Check sheet for the drawn part. Datum: minimum x, y, z corner. Units: mm. Give positions to 0.01 mm unless a question says otherwise; leave off trailing zeros. Write each loop counter-clockwise with the first axis right and the second up, starting at its lowest first coordinate (ties: lowest second). Pieces come first, ordered by that corner, then holes. Notation, with made-up numbers: (65.5, -22) - (115.5, -22) arc R15 cw to (115.5, -6) - close; hole circle Ø6 at (-31.5, -17). An arc over 180 degrees is marked (long way). Use a Markdown table: item, result.
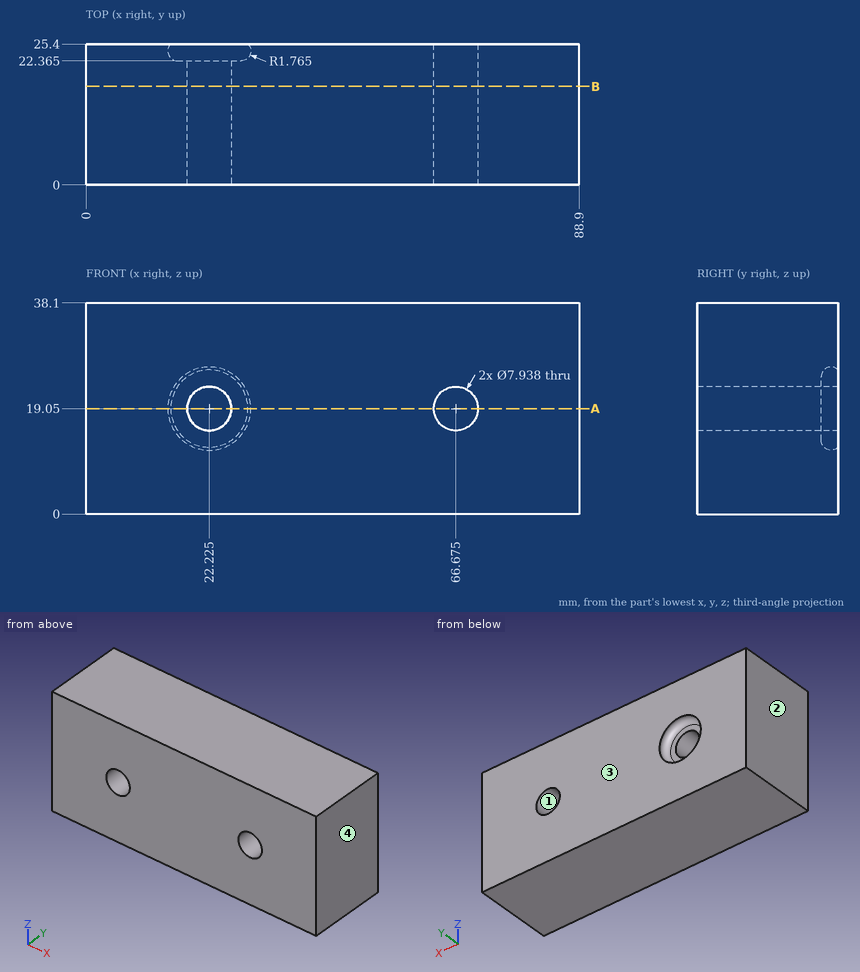
1) Section check B-B on y = 17.75. Count the separate pieces of the cut face and the enclosed holes in it, then the cut area to 3 significant figures.
Working result:
| item | result |
|---|---|
| separate pieces | 1 |
| enclosed holes | 2 |
| area | 3,290 mm² |
2) Material ranges on L1, parallel to X at y = 10.5, z = 15.5; L2, parallel to X at y = 8, z = 17 (1 decimal); L3, parallel to Z at x = 68.5, y = 15.75 (1 decimal), recorded low to high. Write a range as from..to.
Working result:
| item | result |
|---|---|
| L1 | x = 0..20.45, 24..64.9, 68.45..88.9 |
| L2 | x = 0..18.8, 25.6..63.3, 70.1..88.9 |
| L3 | z = 0..15.5, 22.6..38.1 |
3) Section check A-A on z = 19.05. Record the boundary of the cut face in (x, y) (1 decimal), then the cut area to 4 significant figures.
Working result:
| item | result |
|---|---|
| outline | (0, 0) - (18.3, 0) - (18.3, 22.4) - (16.5, 22.4) arc R1.8 cw to (15.3, 25.4) - (0, 25.4) - close; (26.2, 0) - (62.7, 0) - (62.7, 25.4) - (29.2, 25.4) arc R1.8 cw to (28, 22.4) - (26.2, 22.4) - close; (70.6, 0) - (88.9, 0) - (88.9, 25.4) - (70.6, 25.4) - close |
| area | 1,835 mm² |
4) Depth check by flat-ended pin: P1, Ø7, axis at x = 22.225, z = 19.05, coming from the +Y side. Enter the tip coordinate at first touch or a pass-through.
Working result:
| item | result |
|---|---|
| P1 | passes through |
5) Mould release check, pull along X, two halves, no side actions. Record for the marked faces 1, 2, 3 and 4: pulls with the +X half, pulls with the -X half, needs draft (parallel to the pull), parting line crosses it, or undercut.
Working result:
| item | result |
|---|---|
| face 1 | undercut |
| face 2 | pulls with the -X half |
| face 3 | needs draft |
| face 4 | pulls with the +X half |
